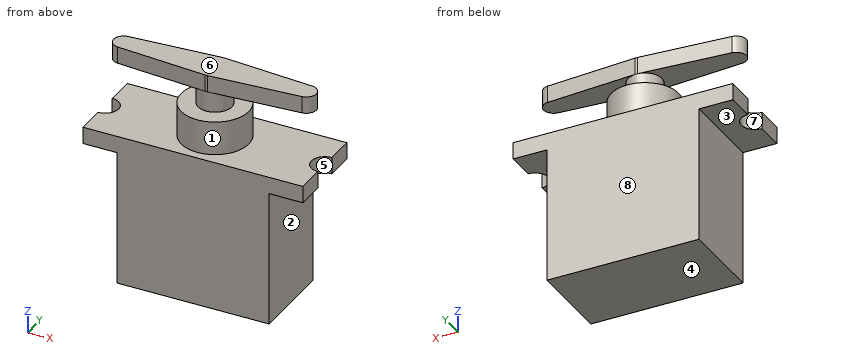
```python
from build123d import *

# Parameters (mm, degrees)
F0_W     = 22.5
F0_H     = 12.5
F1_DEPTH = 20
F3_DEPTH = 2.5
F6_R     = 1.47809988
F7_DEPTH = 2.5


with BuildPart() as f1:
    # F0 (on Top) → F1 (new body)
    with BuildSketch(Plane.XY):
        Rectangle(F0_W, F0_H)
    extrude(amount=F1_DEPTH)

    # F2 (on face) → F3 (join)
    with BuildSketch(Plane.XY.offset(20)):
        with BuildLine():
            Line((16.25, 2), (16.25, 6.25))
            Line((16.25, 6.25), (-16.25, 6.25))
            Line((-16.25, 6.25), (-16.25, 2))
            ThreePointArc((-16.25, 2), (-14.25, 0), (-16.25, -2))
            Line((-16.25, -2), (-16.25, -6.25))
            Line((-16.25, -6.25), (16.25, -6.25))
            Line((16.25, -6.25), (16.25, -2))
            ThreePointArc((16.25, -2), (14.25, 0), (16.25, 2))
        make_face()
    extrude(amount=F3_DEPTH)

    # F4 (on Front) → F5 (revolve)
    with BuildSketch(Plane.XZ):
        Polygon((0, 22.5), (5, 22.5), (5, 27.5), (2.5, 27.5), (2.5, 30.5), (0, 30.5), align=None)
    revolve(axis=Axis((0, 0, 26.5), (0, 0, 1)))

    # F6 (on face) → F7 (join)
    with BuildSketch(Plane.XY.offset(30.5)):
        with BuildLine():
            Line((0.1851851852, -2.4931318552), (13.6111111111, -1.4958791131))
            ThreePointArc((13.6111111111, -1.4958791131), (15, 0), (13.6111111111, 1.4958791131))
            Line((13.6111111111, 1.4958791131), (0.1851851852, 2.4931318552))
            ThreePointArc((0.1851851852, 2.4931318552), (1.832070272, 1.7010345436), (2.5, 0))
            ThreePointArc((2.5, 0), (1.832070272, -1.7010345436), (0.1851851852, -2.4931318552))
        make_face()
        with BuildLine():
            ThreePointArc((-0.1851851852, -2.4931318552), (0, -2.5), (0.1851851852, -2.4931318552))
            ThreePointArc((0.1851851852, -2.4931318552), (1.832070272, -1.7010345436), (2.5, 0))
            ThreePointArc((2.5, 0), (1.832070272, 1.7010345436), (0.1851851852, 2.4931318552))
            ThreePointArc((0.1851851852, 2.4931318552), (0, 2.5), (-0.1851851852, 2.4931318552))
            ThreePointArc((-0.1851851852, 2.4931318552), (-2.5, 0), (-0.1851851852, -2.4931318552))
        make_face()
        Circle(F6_R, mode=Mode.SUBTRACT)
        with BuildLine():
            Line((-13.6111111111, -1.4958791131), (-0.1851851852, -2.4931318552))
            ThreePointArc((-0.1851851852, -2.4931318552), (-2.5, 0), (-0.1851851852, 2.4931318552))
            Line((-0.1851851852, 2.4931318552), (-13.6111111111, 1.4958791131))
            ThreePointArc((-13.6111111111, 1.4958791131), (-15, 0), (-13.6111111111, -1.4958791131))
        make_face()
        Circle(F6_R)
    extrude(amount=F7_DEPTH)


solid = f1.part
```
Geometry: final body of the model. Coordinates: model frame, mm. Face numbers are marked on the shaded views. A direction names the side the tool comes from. Coordinates: 2 decimals unless noted, no trailing zeros. Write each loop counter-clockwise with the first axis right and the second up, starting at its lowest first coordinate (ties: lowest second). Pieces come first, ordered by that corner, then holes. Notation, with made-up numbers: M -1.5,55 L 47.5,55 A21 cw 47.5,79 Z; hole C -11,75 d11. An arc over 180 degrees is marked long. Use CSV: the item, a comma, the result in double quotes. Start each with the question number.
1. Cut plane A-A on x = 6. Return the cut outline in (y, z), plus the area to 3 significant figures.
2. Cut plane B-B on y = 0. Return the cut outline in (x, z).
3. Mould query, pull axis Y, two halves, no side actions, for the marked faces 6, 7 and 8. Classes: pulls with the +Y half, pulls with the -Y half, needs draft (parallel to the pull), parting line crosses it, or undercut.
4. Cut plane D-D on x = -2. Return the cut outline in (y, z).
5. Cut plane C-C on z = 30. Return the cut outline in (x, y).
6. Ray query, probe 1 along Z at (x, y) = (11, 1.25); probe 2 along Z at (x, y) = (2.5, -1.75); probe 3 along X at (y, z) = (5.75, 10). Return the intervals inside material, ascending.
7. Reachability of the marked faces 1, 2, 3, 4 and 5 from +Z, -Z, +X, -X, +Y, -Y: full face, straight path, thin tool, end or side. Return the list, or none.
Entries:
1,outline,"M -6.25,0 L 6.25,0 L 6.25,22.5 L -6.25,22.5 Z; M -2.06,30.5 L 2.06,30.5 L 2.06,33 L -2.06,33 Z"
1,area,"292 mm²"
2,outline,"M -15,30.5 L -2.5,30.5 L -2.5,27.5 L -5,27.5 L -5,22.5 L -14.25,22.5 L -14.25,20 L -11.25,20 L -11.25,0 L 11.25,0 L 11.25,20 L 14.25,20 L 14.25,22.5 L 5,22.5 L 5,27.5 L 2.5,27.5 L 2.5,30.5 L 15,30.5 L 15,33 L -15,33 Z"
3,face 6,"needs draft"
3,face 7,"undercut"
3,face 8,"pulls with the +Y half"
4,outline,"M -6.25,0 L 6.25,0 L 6.25,22.5 L 4.58,22.5 L 4.58,27.5 L 1.5,27.5 L 1.5,30.5 L 2.36,30.5 L 2.36,33 L -2.36,33 L -2.36,30.5 L -1.5,30.5 L -1.5,27.5 L -4.58,27.5 L -4.58,22.5 L -6.25,22.5 Z"
5,outline,"C 0,0 d5"
6,probe 1,"0 to 22.5, 30.5 to 33"
6,probe 2,"0 to 27.5, 30.5 to 33"
6,probe 3,"-11.25 to 11.25"
7,face 1,"none"
7,face 2,"-Z, +X, +Y, -Y"
7,face 3,"-Z, -X, +Y, -Y"
7,face 4,"-Z, +X, -X, +Y, -Y"
7,face 5,"-Z, +X"
